For this review, take the finished solid that the model builds, in its own axes (mm). Coordinates: 2 decimals unless noted, no trailing zeros. Loops run counter-clockwise (first coordinate to the right, second up) from the corner with the lowest first, then second, coordinate; pieces in that order, holes last. Notation, with made-up numbers: M -38.5,-5.75 L 8.5,-5.75 A22 ccw 8.5,2.25 Z; hole C 75,43 d10. An arc over 180 degrees is marked long. Use one line per item in the form item = value.
Autodesk Inventor part; units mm, degrees
ref_plane "YZ Plane" through (0, 0, 0) normal (1, 0, 0) x (0, 1, 0)
ref_plane "XZ Plane" through (0, 0, 0) normal (0, 1, 0) x (-1, 0, 0)
ref_plane "XY Plane" through (0, 0, 0) normal (0, 0, 1) x (1, 0, 0)
sketch "Sketch1" plane through (0, 0, 0) normal (0, 1, 0) x (-1, 0, 0)
  line L0 (8.89, 0) -> (-8.89, 0) construction
  line L1 (8.89, 1.5875) -> (-8.89, 1.5875)
  line L2 (-8.89, -1.5875) -> (8.89, -1.5875)
  arc A0 (8.89, -1.5875) -> (8.89, 1.5875) centre (8.89, 0) ccw
  arc A1 (-8.89, 1.5875) -> (-8.89, -1.5875) centre (-8.89, 0) ccw
  line L3 (8.89, -5.0038) -> (-8.89, -5.0038) construction
  line L4 (8.89, -3.4163) -> (-8.89, -3.4163)
  line L5 (-8.89, -6.5913) -> (8.89, -6.5913)
  arc A2 (8.89, -6.5913) -> (8.89, -3.4163) centre (8.89, -5.0038) ccw
  arc A3 (-8.89, -3.4163) -> (-8.89, -6.5913) centre (-8.89, -5.0038) ccw
  line L6 (8.89, -10.0076) -> (-8.89, -10.0076) construction
  line L7 (8.89, -8.4201) -> (-8.89, -8.4201)
  line L8 (-8.89, -11.5951) -> (8.89, -11.5951)
  arc A4 (8.89, -11.5951) -> (8.89, -8.4201) centre (8.89, -10.0076) ccw
  arc A5 (-8.89, -8.4201) -> (-8.89, -11.5951) centre (-8.89, -10.0076) ccw
  line L9 (12.7, 20.1549) -> (-12.7, 20.1549)
  line L10 (-12.7, 20.1549) -> (-12.7, -17.9451)
  line L11 (-12.7, -17.9451) -> (12.7, -17.9451)
  line L12 (12.7, -17.9451) -> (12.7, 20.1549)
  line L13 (6.35, 13.8049) -> (-6.35, 13.8049) construction
  line L14 (-8.89, -16.5989) -> (8.89, -16.5989)
  arc A6 (8.89, -16.5989) -> (8.89, -13.4239) centre (8.89, -15.0114) ccw
  line L15 (8.89, -13.4239) -> (-8.89, -13.4239)
  line L16 (8.89, -15.0114) -> (-8.89, -15.0114) construction
  arc A7 (-8.89, -13.4239) -> (-8.89, -16.5989) centre (-8.89, -15.0114) ccw
  point P0 (0, 0)
  point P1 (0, -5.0038)
  point P2 (0, -10.0076)
  point P3 (10.4775, -5.0038)
  point P4 (10.4775, 0)
  point P5 (10.4775, -10.0076)
  point P6 (0, -17.9451)
  point P7 (0, -11.5951)
  point P8 (0, 13.8049)
  point P9 (0, 20.1549)
  point P10 (0, -16.5989)
  point P11 (10.4775, -15.0114)
  dimension "d1" = 17.78
  dimension "d3" = 3.175
  dimension "d4" = 5.0038
  dimension "d5" = 5.0038
  dimension "d8" = 25.4
  dimension "d9" = 38.1
  dimension "d10" = 6.35
  dimension "d11" = 12.7
  dimension "d12" = 6.35
  dimension "d25" = 5.0038
extrude "Extrusion1" add sketch "Sketch1" along normal blind 3.175 contours A0 L2 A1 L1 | A2 L5 A3 L4 | A4 L8 A5 L7 | L12 L11 L10 L9 | A7 L15 A6 L14
hole "Hole1" at (-6.35, 0, 13.8049) at (6.35, 0, 13.8049) direction (0, 1, 0) diameter 5.1054 end through all
fillet "Fillet1" radius 3.175 4 edges at (-12.7, 1.5875, -17.9451) (12.7, 1.5875, -17.9451) (12.7, 1.5875, 20.1549) (-12.7, 1.5875, 20.1549)
properties part number "EL2-035" material "Aluminum 6061"
1. Wall thickness on line 1 along Z through (x, y) = (-6.35, 1.25); line 2 along X through (y, z) = (0.9, 16); line 3 along Z through (x, y) = (-7, 2.25): over which ranges is each line inside the solid? List them lowest first. Write a range as from..to.
Computed values:
line_1 = -17.95..11.25, 16.36..20.15
line_2 = -12.7..-7.65, -5.05..5.05, 7.65..12.7
line_3 = -17.95..11.34, 16.27..20.15
2. For pin 1 Ø8 at (x, z) = (5, 6) entering from -Y, flat-tipped, find the tip position at first contact; note if it passes through.
Computed values:
pin_1 = 0
3. Consider section B-B on y = 0.65. Write out the cut boundary in (x, z) (3 decimals), plus the area to 3 significant figures.
Computed values:
outline = M -12.7,-14.77 A3.175 ccw -9.525,-17.945 L 9.525,-17.945 A3.175 ccw 12.7,-14.77 L 12.7,16.98 A3.175 ccw 9.525,20.155 L -9.525,20.155 A3.175 ccw -12.7,16.98 Z; hole C -6.35,13.805 d5.105; hole C 6.35,13.805 d5.105
area = 918 mm2
4. Draft analysis for pull direction Z (two halves, no side actions). For faces 1 (the face through (11.795, 1.61, -16.99)), 2 (the face through (12.7, 2, 1)), 3 (the face through (11.745, 1.61, 19.25)), 4 (the face through (4.625, 1.61, 15.686)), state which applies: +Z half, -Z half, draft (parallel to the pull), parting line (faces both ways), or undercut.
Computed values:
face_1 = -Z half
face_2 = draft
face_3 = +Z half
face_4 = undercut
5. Consider section A-A on x = 6.35. Write out the cut boundary in (y, z) (3 decimals).
Computed values:
outline = M 0,-17.945 L 3.175,-17.945 L 3.175,11.252 L 0,11.252 Z; M 0,16.358 L 3.175,16.358 L 3.175,20.155 L 0,20.155 Z
